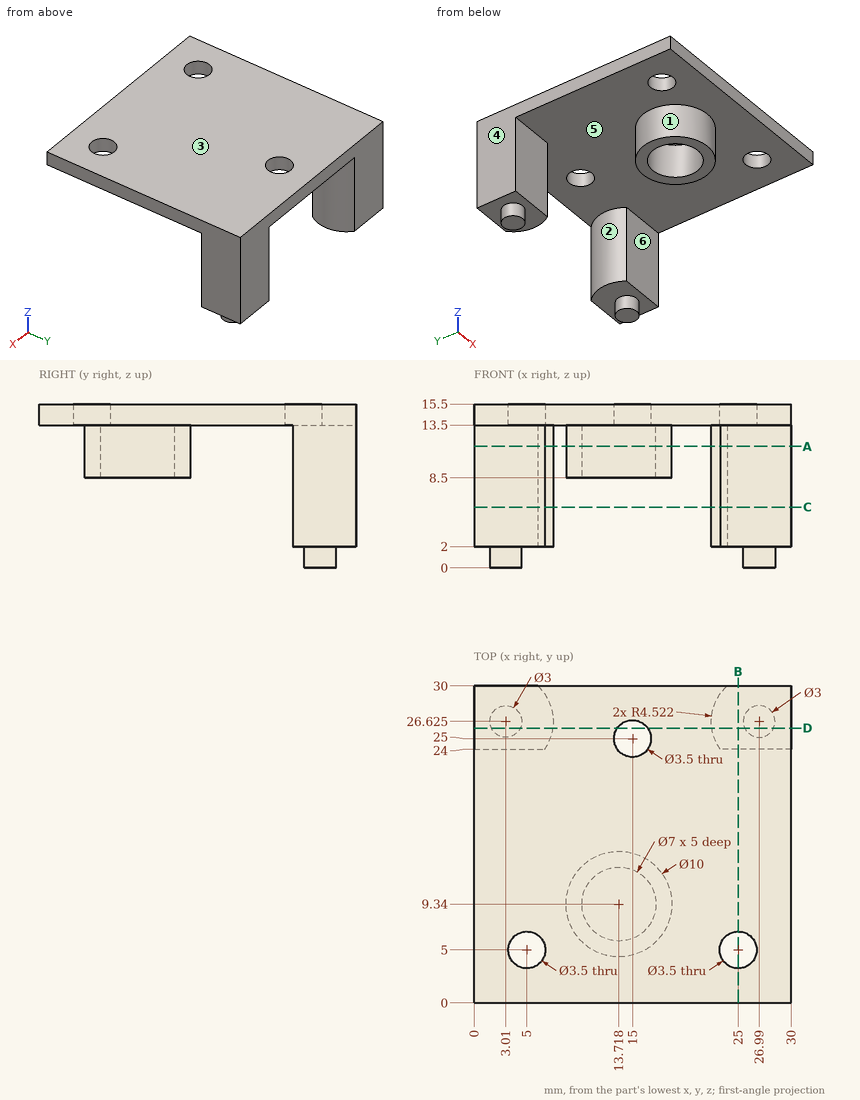
The drawing under review shows one solid part. Ordinate dimensions are in mm from its lowest x, y, z. A direction names the side the tool comes from. Give positions to 0.01 mm unless a question says otherwise; leave off trailing zeros. Loops run counter-clockwise (first coordinate to the right, second up) from the corner with the lowest first, then second, coordinate; pieces in that order, holes last. Notation, with made-up numbers: M 5.25,22 L 24.25,22 A17 ccw 24.25,30 Z; hole C 75.25,34 d3. An arc over 180 degrees is marked long. One line per item, written item: value. Start each with the question number.
Q1. Add section C-C (z = 5.75). Give the boundary of the cut face in (x, y) (1 decimal).
Q2. Add section B-B (x = 25). Give the boundary of the cut face in (y, z), and give its area (3 significant figures).
Q3. Draft analysis for pull direction X (two halves, no side actions). For the marked faces 1, 2 and 3, state which applies: released by +X, released by -X, zero draft, split by the parting line, or undercut.
Q4. Add section A-A (z = 11.5). Give the boundary of the cut face in (x, y) (1 decimal), and give its area (3 significant figures).
Q5. Clearance check with flat-ended pins moving along their axes: pin 1 Ø3.5 at (x, z) = (2.5, 5) entering from -Y; pin 2 Ø3 at (x, y) = (5, 5) entering from +Z; pin 3 Ø11 at (x, y) = (16, 10.5) entering from -Z; pin 4 Ø2 at (x, y) = (12, 8.5) entering from -Z. State where each tip first meets the part, or that it passes through.
Q6. For L1, parallel to Y at x = 15, z = 13.9; L2, parallel to Y at x = 5, z = 15.05; L3, parallel to Z at x = 13.75, y = 28, list the stretches that pass through material, from the lowest coordinate up.
Q7. Machinability: for the marked faces 4, 5 and 6, which of the approach directions +Z, -Z, +X, -X, +Y, -Y give a long, thin tool a straight path to every point of the face, cutting with its end or side? Answer none if there is none.
Q8. Add section D-D (y = 26). Give the boundary of the cut face in (x, z), and give its area (3 significant figures).
Reply:
1. outline: M 0,24 L 6.7,24 A4.5 ccw 6,30 L 0,30 Z; M 23.3,24 L 30,24 L 30,30 L 24,30 A4.5 ccw Z
2. outline: M 0,13.5 L 3.25,13.5 L 3.25,15.5 L 0,15.5 Z; M 6.75,13.5 L 24,13.5 L 24,2 L 30,2 L 30,15.5 L 6.75,15.5 Z
2. area: 122 mm²
3. face 1: split by the parting line
3. face 2: undercut
3. face 3: zero draft
4. outline: M 0,24 L 6.7,24 A4.5 ccw 6,30 L 0,30 Z; C 13.7,9.3 d10; M 23.3,24 L 30,24 L 30,30 L 24,30 A4.5 ccw Z; hole C 13.7,9.3 d7
4. area: 126 mm²
5. pin 1: y = 24
5. pin 2: through
5. pin 3: z = 8.5
5. pin 4: z = 13.5
6. L1: 0 to 23.25, 26.75 to 30
6. L2: 0 to 3.25, 6.75 to 30
6. L3: 13.5 to 15.5
7. face 4: +Z, -Z, -X, +Y, -Y
7. face 5: -Z
7. face 6: -Z, +X, -X, -Y
8. outline: M 0,2 L 1.65,2 L 1.65,0 L 4.37,0 L 4.37,2 L 7.49,2 L 7.49,13.5 L 13.56,13.5 L 13.56,15.5 L 0,15.5 Z; M 16.44,13.5 L 22.51,13.5 L 22.51,2 L 25.63,2 L 25.63,0 L 28.35,0 L 28.35,2 L 30,2 L 30,15.5 L 16.44,15.5 Z
8. area: 237 mm²
